from build123d import *

# Parameters (mm, degrees)
BOSS_EXTRUDE1_DEPTH = 3.2
SKETCH3_R           = 1.05
CUT_EXTRUDE1_DEPTH  = 16.4
EXTRUDE_THIN1_DEPTH = 1.6
FILLET1_R           = 0.65
SKETCH5_W           = 13.579197801
SKETCH5_H           = 3.2
CUT_EXTRUDE2_DEPTH  = 16.4
FILLET2_R           = 0.3
FILLET3_R           = 0.7
LPATTERN1_COUNT     = 2
LPATTERN1_PITCH     = 15.1
LPATTERN2_COUNT     = 2
LPATTERN2_PITCH     = 8.6


with BuildPart() as part:
    # Sketch2 → Boss-Extrude1 (new body, symmetric)
    with BuildSketch(Plane(origin=(0, 0, 0), x_dir=(1, 0, 0), z_dir=(0, 1, 0))):
        Polygon((0, 0), (19.8, 0), (19.8, 9.1), (9.5, 9.1), (9, 11.2), (0, 11.2), align=None)
    extrude(amount=BOSS_EXTRUDE1_DEPTH, both=True)

    # Sketch3 → Cut-Extrude1 (cut)
    with BuildSketch(Plane(origin=(0, 3.2, 0), x_dir=(1, 0, 0), z_dir=(0, 1, 0))):
        with Locations((5.15, 2.35)):
            Circle(SKETCH3_R)
        with Locations((14.65, 2.35)):
            Circle(SKETCH3_R)
    extrude(amount=-CUT_EXTRUDE1_DEPTH, mode=Mode.SUBTRACT)

    # Sketch4 → Extrude-Thin1 (add, symmetric)
    with BuildSketch(Plane(origin=(0, 0, 0), x_dir=(1, 0, 0), z_dir=(0, 1, 0))):
        with BuildLine():
            Line((1.292236799, 10.001697091), (25.025910468, 12.027810166))
            ThreePointArc((25.025910468, 12.027810166), (27.942123478, 15.488402844), (31.402716155, 12.572189834))
            Line((31.402716155, 12.572189834), (31.0041658, 12.538166105))
            ThreePointArc((31.0041658, 12.538166105), (27.776970564, 15.065633982), (25.487099181, 11.665726334))
            Line((25.487099181, 11.665726334), (1.326260528, 9.603146736))
            Line((1.326260528, 9.603146736), (1.292236799, 10.001697091))
        make_face()
    extrude(amount=EXTRUDE_THIN1_DEPTH, both=True)

    # Fillet1
    fillet1_edges = [part.edges().sort_by_distance(p)[0] for p in [
        (19.8, 3.2, -4.55),
        (0, 0, -11.2),
        (9, 0, -11.2),
        (9.5, 0, -9.1),
        (19.8, 0, -9.1),
        (14.65, 3.2, -9.1),
        (9.25, 3.2, -10.15),
        (4.5, 3.2, -11.2),
        (0, 3.2, -5.6),
        (4.5, -3.2, -11.2),
        (9.25, -3.2, -10.15),
        (14.65, -3.2, -9.1),
        (19.8, -3.2, -4.55),
        (0, -3.2, -5.6),
    ]]
    fillet(fillet1_edges, radius=FILLET1_R)

    # Sketch5 → Cut-Extrude2 (cut)
    with BuildSketch(Plane(origin=(-0.838304969, 0, -9.819815492), x_dir=(-0.996375889, 0, 0.085059323), z_dir=(-0.085059323, 0, -0.996375889))):
        with Locations((-4.790866227, 0)):
            Rectangle(SKETCH5_W, SKETCH5_H)
    extrude(amount=CUT_EXTRUDE2_DEPTH, mode=Mode.SUBTRACT)

    # Fillet2
    fillet2_edges = [part.edges().sort_by_distance(p)[0] for p in [
        (25.025910468, 0, -12.027810166),
    ]]
    fillet(fillet2_edges, radius=FILLET2_R)

    # Fillet3
    fillet3_edges = [part.edges().sort_by_distance(p)[0] for p in [
        (25.487099181, 0, -11.665726334),
    ]]
    fillet(fillet3_edges, radius=FILLET3_R)

    # Sketch6 → Revolve1 (revolve)
    with BuildSketch(Plane(origin=(0, 0, 0), x_dir=(1, 0, 0), z_dir=(0, 1, 0))):
        Polygon((2.3, 0.658981297), (2.3, -2.4), (3.7, -2.4), (3.7, -1.7), (2.95, -1.7), (2.95, -0.1), (4.2, -0.1), (4.2, 0.658981297), align=None)
    revolve1 = revolve(axis=Axis((2.3, 0, -0.658981297), (0, 0, 1)))

    # LPattern1: Revolve1 ×2
    with Locations(*[(i * LPATTERN1_PITCH, 0, 0) for i in range(1, LPATTERN1_COUNT)]):
        add(revolve1)

    # LPattern2: Revolve1 ×2
    with Locations(*[(i * LPATTERN2_PITCH, 0, 0) for i in range(1, LPATTERN2_COUNT)]):
        add(revolve1)


solid = part.part
Input: part model. Units: mm. Frame: model coordinates. A direction names the side the tool comes from. Round coordinates to 2 decimals unless told otherwise and drop trailing zeros. Order: outer loops, then holes, each group sorted by start corner. A loop starts at its lowest first (then second) coordinate and runs counter-clockwise, first axis right, second up. Notation, with made-up numbers: (32.5, 50.5) - (44.5, 50.5) arc R14 ccw to (44.5, 60.5) - close; hole circle Ø2 at (74.5, 29). An arc over 180 degrees is marked (long way). Answer as a JSON object with one key per item and string values. Group by question number.
(1) Cut plane A-A (z = -2.35). Return loops of the section in (x, y), then the cut area to 3 significant figures.
(2) Pin query (flat end, axial travel): P1, Ø1.3, axis at x = 5.15, z = -2.35, coming from the -Y side; P2, Ø3, axis at x = 2.5, y = 0.5, coming from the -Z side; P3, Ø1.5, axis at y = 0, z = -6.5, coming from the +X side; P4, Ø3, axis at x = 18, y = -0.5, coming from the -Z side. Return the tip coordinate at first contact, or that it passes through.
(3) Material intervals for probe 1 along X at (y, z) = (1.5, -2.35); probe 2 along Z at (x, y) = (14.65, 0.25); probe 3 along X at (y, z) = (1.25, -1.75), sorted ascending. Write a range as from..to.
(4) Cut plane D-D (y = 0). Count the separate pieces of the cut face and the enclosed holes in it, then the cut area to 3 significant figures.
(5) Reachability of faces 4 (the face through (10.25, 0.03, 0.89)), 5 (the face through (19.8, 0, -4)), 6 (the face through (9.5, 0.06, 2.05)) from +Z, -Z, +X, -X, +Y, -Y: full face, straight path, thin tool, end or side. Return the list, or none.
(6) Draft query along Z for faces 1 (the face through (9.068, 3.005, -10.115)), 2 (the face through (3, -1, 1.7)), 3 (the face through (0, 0, -5)). Return one class per face: released by +Z, released by -Z, zero draft, split by the parting line, or undercut.
(7) Cut plane B-B (x = 14.65). Return loops of the section in (y, z), then the cut area to 3 significant figures.
(8) Cut plane C-C (x = 10.9). Return loops of the section in (y, z), then the cut area to 3 significant figures.
Here are the results:
{
 "1": {"outline": "(0, -2.55) arc R0.65 ccw to (0.65, -3.2) - (4.1, -3.2) - (4.1, 3.2) - (0.65, 3.2) arc R0.65 ccw to (0, 2.55) - close; (6.2, -3.2) - (13.6, -3.2) - (13.6, 3.2) - (6.2, 3.2) - close; (15.7, -3.2) - (19.15, -3.2) arc R0.65 ccw to (19.8, -2.55) - (19.8, 2.55) arc R0.65 ccw to (19.15, 3.2) - (15.7, 3.2) - close", "area": "99.5 mm^2"},
 "2": {"P1": "passes through", "P2": "stops at z = -11.2", "P3": "stops at x = 19.8", "P4": "stops at z = -11.56"},
 "3": {"probe 1": "x = 0..4.1, 6.2..13.6, 15.7..19.8", "probe 2": "z = -11.14..-10.74, -9.1..-3.4, -1.3..0", "probe 3": "x = 0..4.29, 6.01..13.79, 15.51..19.8"},
 "4": {"separate pieces": "1", "enclosed holes": "2", "area": "208 mm^2"},
 "5": {"face 4": "none", "face 5": "+Z, +X, +Y, -Y", "face 6": "+Z"},
 "6": {"face 1": "released by -Z", "face 2": "undercut", "face 3": "zero draft"},
 "7": {"outline": "(-3.2, -8.45) arc R0.65 ccw to (-2.55, -9.1) - (2.55, -9.1) arc R0.65 ccw to (3.2, -8.45) - (3.2, -3.4) - (-3.2, -3.4) - close; (-3.2, -1.3) - (3.2, -1.3) - (3.2, 0) - (-3.2, 0) - close; (-1.6, -11.14) - (1.6, -11.14) - (1.6, -10.74) - (-1.6, -10.74) - close", "area": "45.9 mm^2"},
 "8": {"outline": "(-3.2, -8.45) arc R0.65 ccw to (-2.55, -9.1) - (2.55, -9.1) arc R0.65 ccw to (3.2, -8.45) - (3.2, 0) - (1.9, 0) - (1.9, 0.1) - (0.65, 0.1) - (0.65, 1.7) - (1.4, 1.7) - (1.4, 2.4) - (-1.4, 2.4) - (-1.4, 1.7) - (-0.65, 1.7) - (-0.65, 0.1) - (-1.9, 0.1) - (-1.9, 0) - (-3.2, 0) - close; (-1.6, -10.82) - (1.6, -10.82) - (1.6, -10.42) - (-1.6, -10.42) - close", "area": "63.8 mm^2"}
}
